Verification items for the finished model (mm, model axes). A direction names the side the tool comes from. Give positions to 0.01 mm unless a question says otherwise; leave off trailing zeros. Write each loop counter-clockwise with the first axis right and the second up, starting at its lowest first coordinate (ties: lowest second). Pieces come first, ordered by that corner, then holes. Notation, with made-up numbers: (81, 84.5) - (88, 84.5) arc R17 cw to (88, 103.5) - close; hole circle Ø7 at (57, -20.75). An arc over 180 degrees is marked (long way). Put each result on its own line as item: value.
from build123d import *

# Parameters (mm, degrees)
SKETCH1_R           = 24.5
BOSS_EXTRUDE1_DEPTH = 20
SLOT_DEPTH          = 41.006249512
SKETCH4_R           = 0.5
RELIEFS_DEPTH       = 41.006249512
FILLET1_R           = 0.25
CIRPATTERN1_DEPTH   = 20


# Read off the part's stored shape, not the designer's step: CirPattern1
with BuildPart() as part:
    # Sketch1 → Boss-Extrude1 (new body)
    with BuildSketch(Plane(origin=(0, 0, 0), x_dir=(1, 0, 0), z_dir=(0, 1, 0))):
        with Locations(Location((0, 0, 0), (0, 0, 270))):
            Circle(SKETCH1_R)
        with BuildLine():
            Line((2.02, -5.660362179), (2.02, -7.55))
            Line((2.02, -7.55), (-2.02, -7.55))
            Line((-2.02, -7.55), (-2.02, -5.660362179))
            ThreePointArc((-2.02, -5.660362179), (0, 6.01), (2.02, -5.660362179))
        make_face(mode=Mode.SUBTRACT)
    extrude(amount=BOSS_EXTRUDE1_DEPTH)

    # Sketch3 → Slot (cut, through all)
    with BuildSketch(Plane(origin=(0, 20, 0), x_dir=(1, 0, 0), z_dir=(0, 1, 0))):
        with BuildLine():
            Line((0.75, 22.40473751), (0.75, 24.5))
            Line((0.75, 24.5), (-0.75, 24.5))
            Line((-0.75, 24.5), (-0.75, 22.40473751))
            ThreePointArc((-0.75, 22.40473751), (0, 16.5), (0.75, 22.40473751))
        make_face()
    extrude(amount=-SLOT_DEPTH, mode=Mode.SUBTRACT)

    # Sketch4 → Reliefs (cut, through all)
    with BuildSketch(Plane(origin=(0, 20, 0), x_dir=(1, 0, 0), z_dir=(0, 1, 0))):
        with Locations((2.02, -7.55)):
            Circle(SKETCH4_R)
        with Locations((-2.02, -7.55)):
            Circle(SKETCH4_R)
    extrude(amount=-RELIEFS_DEPTH, mode=Mode.SUBTRACT)

    # Fillet1
    fillet1_edges = [part.edges().sort_by_distance(p)[0] for p in [
        (0.75, 10, -24.488517717),
        (-0.75, 10, -24.488517717),
        (-2.02, 10, 5.660362179),
        (2.02, 10, 5.660362179),
    ]]
    fillet(fillet1_edges, radius=FILLET1_R)

    # CirPattern1 outline → CirPattern1 (cut)
    with BuildSketch(Plane(origin=(0, 0, 0), x_dir=(1, 0, 0), z_dir=(0, 1, 0))):
        with BuildLine():
            ThreePointArc((-12.270617331, 21.205705608), (-12.075969293, 21.229484159), (-11.924042943, 21.10550165))
            Line((-11.924042943, 21.10550165), (-11.076092704, 19.489867452))
            ThreePointArc((-11.076092704, 19.489867452), (-7.66793234, 14.610024423), (-9.747908665, 20.18695221))
            Line((-9.747908665, 20.18695221), (-10.595858905, 21.802586408))
            ThreePointArc((-10.595858905, 21.802586408), (-10.611590506, 21.998049435), (-10.481448454, 22.144733873))
            ThreePointArc((-10.481448454, 22.144733873), (-11.385717715, 21.693672628), (-12.270617331, 21.205705608))
        make_face()
        with BuildLine():
            ThreePointArc((11.924042943, 21.10550165), (12.075969293, 21.229484159), (12.270617331, 21.205705608))
            ThreePointArc((12.270617331, 21.205705608), (11.385717715, 21.693672628), (10.481448454, 22.144733873))
            ThreePointArc((10.481448454, 22.144733873), (10.611590506, 21.998049435), (10.595858905, 21.802586408))
            Line((10.595858905, 21.802586408), (9.747908665, 20.18695221))
            ThreePointArc((9.747908665, 20.18695221), (7.66793234, 14.610024423), (11.076092704, 19.489867452))
            Line((11.076092704, 19.489867452), (11.924042943, 21.10550165))
        make_face()
        with BuildLine():
            ThreePointArc((20.366431348, 13.14661455), (20.558572994, 13.185791915), (20.719874829, 13.0742796))
            ThreePointArc((20.719874829, 13.0742796), (20.163104714, 13.917586295), (19.572032661, 14.737216071))
            ThreePointArc((19.572032661, 14.737216071), (19.619100068, 14.546853424), (19.514334228, 14.381090349))
            Line((19.514334228, 14.381090349), (18.01268893, 13.344579438))
            ThreePointArc((18.01268893, 13.344579438), (13.579233788, 9.37306832), (18.86478605, 12.11010364))
            Line((18.86478605, 12.11010364), (20.366431348, 13.14661455))
        make_face()
        with BuildLine():
            ThreePointArc((24.143115774, 2.175996491), (24.331455382, 2.121393649), (24.422458706, 1.947693698))
            ThreePointArc((24.422458706, 1.947693698), (24.321367415, 2.953148666), (24.178900053, 3.95357967))
            ThreePointArc((24.178900053, 3.95357967), (24.132110239, 3.763148603), (23.962310754, 3.665059802))
            Line((23.962310754, 3.665059802), (22.150979237, 3.445124337))
            ThreePointArc((22.150979237, 3.445124337), (16.379696423, 1.988855222), (22.331784258, 1.956061026))
            Line((22.331784258, 1.956061026), (24.143115774, 2.175996491))
        make_face()
        with BuildLine():
            ThreePointArc((22.388903332, -9.293116141), (22.530294567, -9.428990336), (22.530151616, -9.625085358))
            ThreePointArc((22.530151616, -9.625085358), (22.907897946, -8.687819733), (23.246672831, -7.735774188))
            ThreePointArc((23.246672831, -7.735774188), (23.116744778, -7.882648213), (22.920810662, -7.890591777))
            Line((22.920810662, -7.890591777), (21.21474715, -7.243567232))
            ThreePointArc((21.21474715, -7.243567232), (15.427768004, -5.850980635), (20.682839819, -8.646091596))
            Line((20.682839819, -8.646091596), (22.388903332, -9.293116141))
        make_face()
        with BuildLine():
            ThreePointArc((15.505662952, -18.633287859), (15.567714786, -18.819306267), (15.476458308, -18.992873354))
            ThreePointArc((15.476458308, -18.992873354), (16.246505127, -18.33851333), (16.988913016, -17.652955405))
            ThreePointArc((16.988913016, -17.652955405), (16.805611676, -17.722625319), (16.628429074, -17.638603872))
            Line((16.628429074, -17.638603872), (15.418472156, -16.272844842))
            ThreePointArc((15.418472156, -16.272844842), (10.941523861, -12.350427345), (14.295706033, -17.26752883))
            Line((14.295706033, -17.26752883), (15.505662952, -18.633287859))
        make_face()
        with BuildLine():
            ThreePointArc((5.070262053, -23.704797884), (5.038759159, -23.89834593), (4.877294914, -24.009622953))
            ThreePointArc((4.877294914, -24.009622953), (5.863233775, -23.788074527), (6.839197968, -23.52605728))
            ThreePointArc((6.839197968, -23.52605728), (6.644515468, -23.502562546), (6.526674779, -23.345824387))
            Line((6.526674779, -23.345824387), (6.090011003, -21.574209808))
            ThreePointArc((6.090011003, -21.574209808), (3.948708458, -16.020539989), (4.633598277, -21.933183305))
            Line((4.633598277, -21.933183305), (5.070262053, -23.704797884))
        make_face()
        with BuildLine():
            ThreePointArc((-6.526674779, -23.345824387), (-6.644515468, -23.502562546), (-6.839197968, -23.52605728))
            ThreePointArc((-6.839197968, -23.52605728), (-5.863233775, -23.788074527), (-4.877294914, -24.009622953))
            ThreePointArc((-4.877294914, -24.009622953), (-5.038759159, -23.89834593), (-5.070262053, -23.704797884))
            Line((-5.070262053, -23.704797884), (-4.633598277, -21.933183305))
            ThreePointArc((-4.633598277, -21.933183305), (-3.948708458, -16.020539989), (-6.090011003, -21.574209808))
            Line((-6.090011003, -21.574209808), (-6.526674779, -23.345824387))
        make_face()
        with BuildLine():
            ThreePointArc((-16.628429074, -17.638603872), (-16.805611676, -17.722625319), (-16.988913016, -17.652955405))
            ThreePointArc((-16.988913016, -17.652955405), (-16.246505127, -18.33851333), (-15.476458308, -18.992873354))
            ThreePointArc((-15.476458308, -18.992873354), (-15.567714786, -18.819306267), (-15.505662952, -18.633287859))
            Line((-15.505662952, -18.633287859), (-14.295706033, -17.26752883))
            ThreePointArc((-14.295706033, -17.26752883), (-10.941523861, -12.350427345), (-15.418472156, -16.272844842))
            Line((-15.418472156, -16.272844842), (-16.628429074, -17.638603872))
        make_face()
        with BuildLine():
            ThreePointArc((-22.920810662, -7.890591777), (-23.116744778, -7.882648213), (-23.246672831, -7.735774188))
            ThreePointArc((-23.246672831, -7.735774188), (-22.907897946, -8.687819733), (-22.530151616, -9.625085358))
            ThreePointArc((-22.530151616, -9.625085358), (-22.530294567, -9.428990336), (-22.388903332, -9.293116141))
            Line((-22.388903332, -9.293116141), (-20.682839819, -8.646091596))
            ThreePointArc((-20.682839819, -8.646091596), (-15.427768004, -5.850980635), (-21.21474715, -7.243567232))
            Line((-21.21474715, -7.243567232), (-22.920810662, -7.890591777))
        make_face()
        with BuildLine():
            ThreePointArc((-23.962310754, 3.665059802), (-24.132110239, 3.763148603), (-24.178900053, 3.95357967))
            ThreePointArc((-24.178900053, 3.95357967), (-24.321367415, 2.953148666), (-24.422458706, 1.947693698))
            ThreePointArc((-24.422458706, 1.947693698), (-24.331455382, 2.121393649), (-24.143115774, 2.175996491))
            Line((-24.143115774, 2.175996491), (-22.331784258, 1.956061026))
            ThreePointArc((-22.331784258, 1.956061026), (-16.379696423, 1.988855222), (-22.150979237, 3.445124337))
            Line((-22.150979237, 3.445124337), (-23.962310754, 3.665059802))
        make_face()
        with BuildLine():
            ThreePointArc((-19.514334228, 14.381090349), (-19.619100068, 14.546853424), (-19.572032661, 14.737216071))
            ThreePointArc((-19.572032661, 14.737216071), (-20.163104714, 13.917586295), (-20.719874829, 13.0742796))
            ThreePointArc((-20.719874829, 13.0742796), (-20.558572994, 13.185791915), (-20.366431348, 13.14661455))
            Line((-20.366431348, 13.14661455), (-18.86478605, 12.11010364))
            ThreePointArc((-18.86478605, 12.11010364), (-13.579233788, 9.37306832), (-18.01268893, 13.344579438))
            Line((-18.01268893, 13.344579438), (-19.514334228, 14.381090349))
        make_face()
    extrude(amount=CIRPATTERN1_DEPTH, mode=Mode.SUBTRACT)


solid = part.part
Q1. Release check for a two-part mould opening along X. For faces 1 (the face through (-15.387, 9.86, 5.965)), 2 (the face through (-24.33, 9.86, 2.88)), 3 (the face through (24.313, 9.86, 3.021)) record: released by +X, released by -X, zero draft, split by the parting line, or undercut.
Answers follow:
face 1: undercut
face 2: released by -X
face 3: released by +X
Q2. Scan lines: line 1 along Z through (x, y) = (16, 4); line 2 along Z through (x, y) = (0, 11.25); line 3 along Z through (x, y) = (18, 2.25). Record each from-to range of solid material in increasing order.
Answers follow:
line 1: z = -18.55 to -14.08, -8.08 to 4.91, 8.92 to 16.93
line 2: z = -16.5 to -6.01, 7.55 to 24.5
line 3: z = -16.62 to -13.36, -8.8 to -5.03, 0.32 to 3.92, 9.91 to 16.62
Q3. Section check A-A, the plane z = 0. Record the cut outline in (x, y), plus the area to 3 significant figures.
Answers follow:
outline: (-24.5, 0) - (-21.22, 0) - (-21.22, 20) - (-24.5, 20) - close; (-17.49, 0) - (-6.01, 0) - (-6.01, 20) - (-17.49, 20) - close; (6.01, 0) - (17.49, 0) - (17.49, 20) - (6.01, 20) - close; (21.22, 0) - (24.5, 0) - (24.5, 20) - (21.22, 20) - close
area: 590 mm2
Q4. Set-up check for faces 4 (the face through (23.069, 9.86, -3.557)), 5 (the face through (-4.855, 9.86, 22.831)), 6 (the face through (11.5, 9.9, -20.3)): record each of +Z, -Z, +X, -X, +Y, -Y from which the full face is reachable in a straight line by a thin tool's end or side.
Answers follow:
face 4: +X, +Y, -Y
face 5: +Y, -Y
face 6: -Z, +Y, -Y
Q5. Section check B-B, the plane z = -9.5. Record the cut outline in (x, y).
Answers follow:
outline: (-22.58, 0) - (-18.6, 0) - (-18.6, 20) - (-22.58, 20) - close; (-13.5, 0) - (13.5, 0) - (13.5, 20) - (-13.5, 20) - close; (18.6, 0) - (22.58, 0) - (22.58, 20) - (18.6, 20) - close
Q6. Go/stop test with flat-tipped pins: pin 1 Ø2 at (y, z) = (5.5, -23) entering from +X; pin 2 Ø10 at (y, z) = (13.5, 11) entering from -X; pin 3 Ø4 at (y, z) = (14.5, 8.5) entering from -X. Record where each tip stops, or that it passes through.
Answers follow:
pin 1: stops at x = 10.61
pin 2: stops at x = -23.75
pin 3: stops at x = -23.62
Q7. Section check C-C, the plane z = -18. Record the cut outline in (x, y), plus the area to 3 significant figures.
Answers follow:
outline: (-16.62, 0) - (-11.97, 0) - (-11.97, 20) - (-16.62, 20) - close; (-6.15, 0) - (-2.6, 0) - (-2.6, 20) - (-6.15, 20) - close; (2.6, 0) - (6.15, 0) - (6.15, 20) - (2.6, 20) - close; (11.97, 0) - (16.62, 0) - (16.62, 20) - (11.97, 20) - close
area: 328 mm2
